Read the model definition and answer for the solid it produces. Units are mm, in the model's axes. A direction names the side the tool comes from. Coordinates: 2 decimals unless noted, no trailing zeros. Write each loop counter-clockwise with the first axis right and the second up, starting at its lowest first coordinate (ties: lowest second). Pieces come first, ordered by that corner, then holes. Notation, with made-up numbers: M -14.75,87.5 L 4.25,87.5 A19 ccw 4.25,101.5 Z; hole C 10.5,16 d4. An arc over 180 degrees is marked long. Write item = value, one per line.
from build123d import *

# Parameters (mm, degrees)
SKETCH_1_W          = 200
SKETCH_1_H          = 10
EXTRUDE_1_DEPTH     = 200
SKETCH_2_W          = 15
SKETCH_2_H          = 15
EXTRUDE_2_DEPTH     = 133
EXTRUDE_3_REACH     = 309.691
SKETCH_6_W          = 15
SKETCH_6_H          = 15
CUT_EXTRUDE_1_REACH = 318.937
SKETCH_7_W          = 7
SKETCH_7_H          = 7
SKETCH_8_W          = 52
SKETCH_8_H          = 25
EXTRUDE_4_DEPTH     = 60
SKETCH_9_W          = 3
SKETCH_9_H          = 36
EXTRUDE_7_DEPTH     = 47.5
SKETCH_12_W         = 42
SKETCH_12_H         = 42
EXTRUDE_8_DEPTH     = 42
EXTRUDE_9_REACH     = 296.4
SKETCH_14_W         = 36
SKETCH_14_H         = 5
SKETCH_15_W         = 20
SKETCH_15_H         = 8
EXTRUDE_10_DEPTH    = 15
EXTRUDE_11_REACH    = 331.87
SKETCH_13_R         = 3.175


with BuildPart() as part:
    # 草图1 → 凸台-拉伸1 (new body)
    with BuildSketch(Plane.XY):
        with Locations((100, 5)):
            Rectangle(SKETCH_1_W, SKETCH_1_H)
    extrude(amount=-EXTRUDE_1_DEPTH)

    # 草图2 → 凸台-拉伸2 (add)
    with BuildSketch(Plane(origin=(0, 10, 0), x_dir=(1, 0, 0), z_dir=(0, 1, 0))):
        with Locations((7.5, 7.5)):
            Rectangle(SKETCH_2_W, SKETCH_2_H)
        with Locations((192.5, 7.5)):
            Rectangle(SKETCH_2_W, SKETCH_2_H)
        with Locations((192.5, 192.5)):
            Rectangle(SKETCH_2_W, SKETCH_2_H)
        with Locations((7.5, 192.5)):
            Rectangle(SKETCH_2_W, SKETCH_2_H)
    extrude(amount=EXTRUDE_2_DEPTH)

    # 草图6 → 凸台-拉伸3 (add, up to next)
    with BuildSketch(Plane.XY.offset(-185), mode=Mode.PRIVATE) as extrude_3_sk1:
        with Locations((7.5, 135.5)):
            Rectangle(SKETCH_6_W, SKETCH_6_H)
    extrude_3_tool1 = extrude(extrude_3_sk1.sketch, amount=EXTRUDE_3_REACH, mode=Mode.PRIVATE) - part.part
    # 草图6 → 凸台-拉伸3 (add, up to next)
    with BuildSketch(Plane.XY.offset(-185), mode=Mode.PRIVATE) as extrude_3_sk2:
        with Locations((192.5, 135.5)):
            Rectangle(SKETCH_6_W, SKETCH_6_H)
    extrude_3_tool2 = extrude(extrude_3_sk2.sketch, amount=EXTRUDE_3_REACH, mode=Mode.PRIVATE) - part.part
    add(extrude_3_tool1.solids().sort_by_distance((7.5, 135.5, -185))[0])
    add(extrude_3_tool2.solids().sort_by_distance((192.5, 135.5, -185))[0])

    # 草图7 → 切除-拉伸1 (cut, up to next)
    with BuildSketch(Plane.XY, mode=Mode.PRIVATE) as cut_extrude_1_sk1:
        with Locations((11.5, 135.5)):
            Rectangle(SKETCH_7_W, SKETCH_7_H)
    cut_extrude_1_tool1 = extrude(cut_extrude_1_sk1.sketch, amount=-CUT_EXTRUDE_1_REACH, mode=Mode.PRIVATE) & part.part
    # 草图7 → 切除-拉伸1 (cut, up to next)
    with BuildSketch(Plane.XY, mode=Mode.PRIVATE) as cut_extrude_1_sk2:
        with Locations((188.5, 135.5)):
            Rectangle(SKETCH_7_W, SKETCH_7_H)
    cut_extrude_1_tool2 = extrude(cut_extrude_1_sk2.sketch, amount=-CUT_EXTRUDE_1_REACH, mode=Mode.PRIVATE) & part.part
    add(cut_extrude_1_tool1.solids().sort_by_distance((11.5, 135.5, 0))[0], mode=Mode.SUBTRACT)
    add(cut_extrude_1_tool2.solids().sort_by_distance((188.5, 135.5, 0))[0], mode=Mode.SUBTRACT)

    # 草图8 → 凸台-拉伸4 (add)
    with BuildSketch(Plane.XY):
        with Locations((26, 94.5)):
            Rectangle(SKETCH_8_W, SKETCH_8_H)
    extrude(amount=EXTRUDE_4_DEPTH)

    # 草图9 → 凸台-拉伸7 (add)
    with BuildSketch(Plane(origin=(0, 107, 0), x_dir=(1, 0, 0), z_dir=(0, 1, 0))):
        with Locations((50.5, -30)):
            Rectangle(SKETCH_9_W, SKETCH_9_H)
        with Locations((1.5, -30)):
            Rectangle(SKETCH_9_W, SKETCH_9_H)
    extrude(amount=EXTRUDE_7_DEPTH)

    # 草图12 → 凸台-拉伸8 (add)
    with BuildSketch(Plane(origin=(0, 107, 0), x_dir=(1, 0, 0), z_dir=(0, 1, 0))):
        with Locations((26, -33)):
            Rectangle(SKETCH_12_W, SKETCH_12_H)
    extrude(amount=EXTRUDE_8_DEPTH)

    # 草图14 → 凸台-拉伸9 (add, up to next)
    with BuildSketch(Plane.ZY.offset(-49), mode=Mode.PRIVATE) as extrude_9_sk1:
        with Locations((30, 152)):
            Rectangle(SKETCH_14_W, SKETCH_14_H)
    extrude_9_tool1 = extrude(extrude_9_sk1.sketch, amount=EXTRUDE_9_REACH, mode=Mode.PRIVATE) - part.part
    add(extrude_9_tool1.solids().sort_by_distance((49, 152, 30))[0])

    # 草图15 → 凸台-拉伸10 (add)
    with BuildSketch(Plane(origin=(0, 0, -200), x_dir=(-1, 0, 0), z_dir=(0, 0, -1))):
        with Locations((-25, 128)):
            Rectangle(SKETCH_15_W, SKETCH_15_H)
    extrude(amount=-EXTRUDE_10_DEPTH)

    # 草图13 → 凸台-拉伸11 (add, up to next)
    with BuildSketch(Plane(origin=(0, 0, 12), x_dir=(-1, 0, 0), z_dir=(0, 0, -1)), mode=Mode.PRIVATE) as extrude_11_sk1:
        with Locations((-26, 128)):
            Circle(SKETCH_13_R)
    extrude_11_tool1 = extrude(extrude_11_sk1.sketch, amount=EXTRUDE_11_REACH, mode=Mode.PRIVATE) - part.part
    add(extrude_11_tool1.solids().sort_by_distance((26, 128, 12))[0])


solid = part.part
Item 1: Which of the six approach directions +Z, -Z, +X, -X, +Y, -Y give full straight-line access (tool end or side, diameter ignored) to faces 5 (the face through (7, 143, -101)), 6 (the face through (26.41, 131.15, -85.12)), 7 (the face through (30, 150, 48)), 8 (the face through (26, 149, 33))?
Worked answers:
face_5 = -Z, +X, -X, +Y
face_6 = none
face_7 = +Z, +Y
face_8 = +Z, -Z
Item 2: Find section D-D (z = 28). Determine the outline of the cut face in (x, y), and give its area (3 significant figures).
Worked answers:
outline = M 0,82 L 52,82 L 52,154.5 L 0,154.5 Z; hole M 3,107 L 5,107 L 5,149 L 47,149 L 47,107 L 49,107 L 49,149.5 L 3,149.5 Z
area = 3,580 mm²
Item 3: Find section B-B (z = -99). Determine the outline of the cut face in (x, y) (3 decimals), and give its area (3 significant figures).
Worked answers:
outline = M 0,0 L 200,0 L 200,10 L 0,10 Z; M 0,128 L 15,128 L 15,132 L 8,132 L 8,139 L 15,139 L 15,143 L 0,143 Z; C 26,128 d6.35; M 185,128 L 200,128 L 200,143 L 185,143 L 185,139 L 192,139 L 192,132 L 185,132 Z
area = 2,380 mm²
Item 4: Flat-ended cylindrical pins translate along their axes: pin 1 (7.5 mm diameter, centred on x = 192.5, y = 94, fed in from +Z); pin 2 (16.5 mm diameter, centred on x = 11, y = 119.5, fed in from +Z). Find the tip coordinate at first contact, or state that the pin passes through.
Worked answers:
pin_1 = 0
pin_2 = 54
Item 5: Find section A-A (y = 98). Determine the outline of the cut face in (x, z).
Worked answers:
outline = M 0,-200 L 15,-200 L 15,-185 L 0,-185 Z; M 0,-15 L 15,-15 L 15,0 L 52,0 L 52,60 L 0,60 Z; M 185,-200 L 200,-200 L 200,-185 L 185,-185 Z; M 185,-15 L 200,-15 L 200,0 L 185,0 Z
Item 6: Find section C-C (x = 26). Determine the outline of the cut face in (y, z) (3 decimals).
Worked answers:
outline = M 0,-200 L 10,-200 L 10,0 L 0,0 Z; M 82,0 L 107,0 L 107,12 L 124.825,12 L 124.825,-185 L 124,-185 L 124,-200 L 132,-200 L 132,-185 L 131.175,-185 L 131.175,12 L 149,12 L 149,54 L 107,54 L 107,60 L 82,60 Z; M 149.5,12 L 154.5,12 L 154.5,48 L 149.5,48 Z
Item 7: Consider line 1 along Y through (x, z) = (12.5, -62); line 2 along X through (y, z) = (131.5, -51); line 3 along X through (y, z) = (132.5, -48.5). Determine where each line is inside the solid, lowest interval first. Write a range as from..to.
Worked answers:
line_1 = 0..10, 128..132, 139..143
line_2 = 0..15, 185..200
line_3 = 0..8, 192..200
Item 8: For a pull along Z with two mould halves and no side action, classify faces 1 (the face through (192, 68, -185)), 2 (the face through (15, 66, -193)), 3 (the face through (114, 8, 0)), 4 (the face through (10, 72, -185)) as released by +Z, released by -Z, zero draft, split by the parting line, or undercut.
Worked answers:
face_1 = undercut
face_2 = zero draft
face_3 = released by +Z
face_4 = undercut
